Geometry: final body of the model. Coordinates: model frame, mm. Face numbers are marked on the shaded views. A direction names the side the tool comes from. Round coordinates to 2 decimals unless told otherwise and drop trailing zeros. Loops run counter-clockwise (first coordinate to the right, second up) from the corner with the lowest first, then second, coordinate; pieces in that order, holes last. Notation, with made-up numbers: (-13.75, 6.25) - (-4.75, 6.25) arc R12 cw to (-4.75, 25.25) - close; hole circle Ø2 at (-17, 55.25). An arc over 180 degrees is marked (long way). Answer as a JSON object with one key per item and string values. Group by question number.
Item 1: First-contact query: pin 1 (4 mm diameter, centred on x = -77, z = 77, fed in from +Y); pin 2 (15 mm diameter, centred on y = 16.5, z = 73.5, fed in from +X); pin 3 (7.5 mm diameter, centred on x = -77, z = -77, fed in from -Y); pin 4 (6 mm diameter, centred on y = 21.5, z = -54, fed in from -X). Flat tips, straight axial feed; report the tip coordinate or a pass-through.
Item 2: Reachability of the marked faces 5, 6, 7 and 8 from +Z, -Z, +X, -X, +Y, -Y: full face, straight path, thin tool, end or side. Return the list, or none.
Item 3: Section B-B (y = 9.25). Return the cut outline in (x, z).
Item 4: Section A-A (x = 0). Return the cut outline in (y, z).
Item 5: Section C-C (z = -54.5). Return the cut outline in (x, y), plus the area to 3 significant figures.
Item 6: Draft query along Z for the marked faces 1, 2, 3 and 4. Return one class per face: released by +Z, released by -Z, zero draft, split by the parting line, or undercut.
Item 7: Line query: line 1 (X direction, y = 27.5, z = -0.5); line 2 (Z direction, x = -77, y = 12.5); line 3 (X direction, y = 12, z = 77). Output: solid intervals per line, ascending.
Item 8: Section D-D (x = 77). Return the cut outline in (y, z), plus the area to 3 significant figures.
```python
from build123d import *

# Parameters (mm, degrees)
SKETCH1_R           = 100
SKETCH1_W           = 181.371629942
SKETCH1_H           = 180.45561161
BOSS_EXTRUDE1_DEPTH = 30
SKETCH2_R           = 2.28
CUT_EXTRUDE1_DEPTH  = 31
SKETCH3_R           = 97.5
CUT_EXTRUDE2_DEPTH  = 30


with BuildPart() as part:
    # Sketch1 → Boss-Extrude1 (new body)
    with BuildSketch(Plane(origin=(0, 0, 0), x_dir=(1, 0, 0), z_dir=(0, 1, 0))):
        Circle(SKETCH1_R)
        Rectangle(SKETCH1_W, SKETCH1_H)
    extrude(amount=BOSS_EXTRUDE1_DEPTH)

    # Sketch2 → Cut-Extrude1 (cut, through all)
    with BuildSketch(Plane(origin=(0, 30, 0), x_dir=(1, 0, 0), z_dir=(0, 1, 0))):
        with Locations((-77, 77)):
            Circle(SKETCH2_R)
        with Locations((77, 77)):
            Circle(SKETCH2_R)
        with Locations((-77, -77)):
            Circle(SKETCH2_R)
        with Locations((77, -77)):
            Circle(SKETCH2_R)
    extrude(amount=-CUT_EXTRUDE1_DEPTH, mode=Mode.SUBTRACT)

    # Sketch3 → Cut-Extrude2 (cut)
    with BuildSketch(Plane(origin=(0, 0, 0), x_dir=(-1, 0, 0), z_dir=(0, -1, 0))):
        Circle(SKETCH3_R)
    extrude(amount=-CUT_EXTRUDE2_DEPTH, mode=Mode.SUBTRACT)


solid = part.part
```
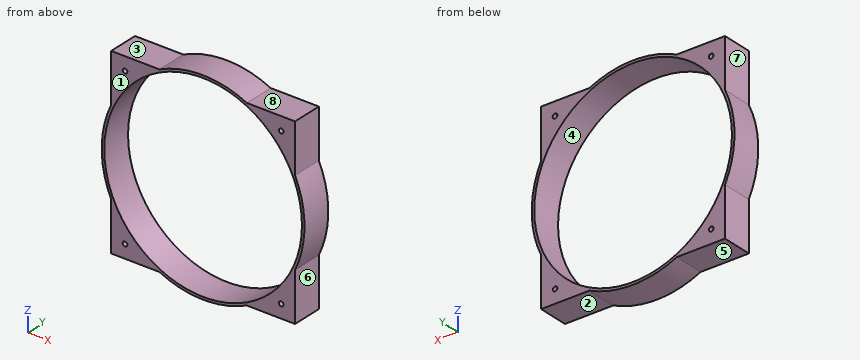
Values:
{
 "1": {"pin 1": "passes through", "pin 2": "stops at x = 90.69", "pin 3": "stops at y = 0", "pin 4": "stops at x = -90.69"},
 "2": {"face 5": "-Z, -X, +Y, -Y", "face 6": "-Z, +X, +Y, -Y", "face 7": "+Z, -X, +Y, -Y", "face 8": "+Z, +X, +Y, -Y"},
 "3": {"outline": "(-90.69, -90.23) - (-43.12, -90.23) arc R100 ccw to (43.12, -90.23) - (90.69, -90.23) - (90.69, -42.14) arc R100 ccw to (90.69, 42.14) - (90.69, 90.23) - (43.12, 90.23) arc R100 ccw to (-43.12, 90.23) - (-90.69, 90.23) - (-90.69, 42.14) arc R100 ccw to (-90.69, -42.14) - close; hole circle Ø195 at (0, 0); hole circle Ø4.56 at (-77, -77); hole circle Ø4.56 at (-77, 77); hole circle Ø4.56 at (77, -77); hole circle Ø4.56 at (77, 77)"},
 "4": {"outline": "(0, -100) - (30, -100) - (30, -97.5) - (0, -97.5) - close; (0, 97.5) - (30, 97.5) - (30, 100) - (0, 100) - close"},
 "5": {"outline": "(-90.69, 0) - (-80.85, 0) - (-80.85, 30) - (-90.69, 30) - close; (80.85, 0) - (90.69, 0) - (90.69, 30) - (80.85, 30) - close", "area": "590 mm^2"},
 "6": {"face 1": "zero draft", "face 2": "released by -Z", "face 3": "released by +Z", "face 4": "undercut"},
 "7": {"line 1": "x = -100 to -97.5, 97.5 to 100", "line 2": "z = -90.23 to -79.28, -74.72 to -59.81, 59.81 to 74.72, 79.28 to 90.23", "line 3": "x = -90.69 to -79.28, -74.72 to -59.81, 59.81 to 74.72, 79.28 to 90.69"},
 "8": {"outline": "(0, -90.23) - (30, -90.23) - (30, -79.28) - (0, -79.28) - close; (0, -74.72) - (30, -74.72) - (30, -59.81) - (0, -59.81) - close; (0, 59.81) - (30, 59.81) - (30, 74.72) - (0, 74.72) - close; (0, 79.28) - (30, 79.28) - (30, 90.23) - (0, 90.23) - close", "area": "1,550 mm^2"}
}
